Could you check a few things on this model? Use its own coordinates, in mm. Face numbers are marked on the shaded views. A direction names the side the tool comes from. Give positions to 0.01 mm unless a question says otherwise; leave off trailing zeros. Write each loop counter-clockwise with the first axis right and the second up, starting at its lowest first coordinate (ties: lowest second). Pieces come first, ordered by that corner, then holes. Notation, with made-up numbers: M 70.25,75 L 102.25,75 A8 ccw 102.25,86 Z; hole C 10.25,-32 d10. An arc over 180 degrees is marked long. One line per item, written item: value.
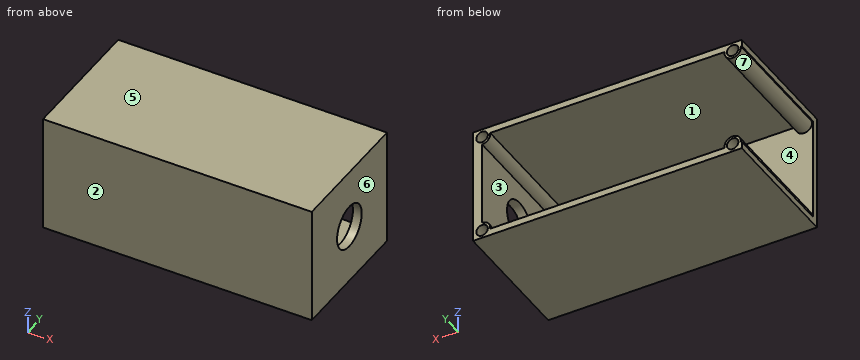
```python
from build123d import *

# Parameters (mm, degrees)
SKETCH1_W                 = 59.28
SKETCH1_H                 = 26
BOSS_EXTRUDE2_DEPTH       = 29
SKETCH3_W                 = 57.28
SKETCH3_H                 = 23
CUT_EXTRUDE1_DEPTH        = 27.5
SKETCH4_R                 = 4.75
SKETCH5_R                 = 4.8654
SKETCH9_R                 = 1.8
BOSS_EXTRUDE4_DEPTH       = 27.5
F_2_0MM_DOWEL_HOLE3_D     = 2.54
F_2_0MM_DOWEL_HOLE3_DEPTH = 10
MIRROR2_COPY_1_SKETCH_R   = 1.8
MIRROR2_COPY_1_DEPTH      = 27.5
MIRROR2_COPY_2_D          = 2.54
MIRROR2_COPY_2_DEPTH      = 10


with BuildPart() as part:
    # Sketch1 → Boss-Extrude2 (new body)
    with BuildSketch(Plane(origin=(0, 0, 0), x_dir=(1, 0, 0), z_dir=(0, 1, 0))):
        with Locations((29.64, 13)):
            Rectangle(SKETCH1_W, SKETCH1_H)
    extrude(amount=BOSS_EXTRUDE2_DEPTH)

    # Sketch3 → Cut-Extrude1 (cut)
    with BuildSketch(Plane(origin=(0, 29, 0), x_dir=(1, 0, 0), z_dir=(0, 1, 0))):
        with Locations((28.64, 13)):
            Rectangle(SKETCH3_W, SKETCH3_H)
    extrude(amount=-CUT_EXTRUDE1_DEPTH, mode=Mode.SUBTRACT)

    # Sketch4 → Cut-Loft1 section 0
    with BuildSketch(Plane(origin=(59.28, 0, 0), x_dir=(0, 0, -1), z_dir=(1, 0, 0))):
        with Locations((13, 14.5)):
            Circle(SKETCH4_R)
    # Sketch5 → Cut-Loft1 section 1
    with BuildSketch(Plane.ZY.offset(-57.28)):
        with Locations((-13, 14.5)):
            Circle(SKETCH5_R)
    loft(mode=Mode.SUBTRACT)

    # Sketch9 → Boss-Extrude4 (add)
    with BuildSketch(Plane(origin=(0, 29, 0), x_dir=(1, 0, 0), z_dir=(0, 1, 0))):
        with Locations((57.28, 1.8)):
            Circle(SKETCH9_R)
    boss_extrude4 = extrude(amount=-BOSS_EXTRUDE4_DEPTH)

    # Ø2.0mm Dowel Hole3
    with Locations(Plane(origin=(0, 29, 0), x_dir=(1, 0, 0), z_dir=(0, 1, 0))):
        with Locations((57.28, 1.8)):
            f_2_0mm_dowel_hole3 = Hole(F_2_0MM_DOWEL_HOLE3_D / 2, depth=F_2_0MM_DOWEL_HOLE3_DEPTH)

    # Mirror1: Boss-Extrude4, Ø2.0mm Dowel Hole3 across plane
    add(boss_extrude4.mirror(Plane(origin=(0, 0, -13), x_dir=(1, 0, 0), z_dir=(0, 0, -1))))
    add(f_2_0mm_dowel_hole3.mirror(Plane(origin=(0, 0, -13), x_dir=(1, 0, 0), z_dir=(0, 0, -1))), mode=Mode.SUBTRACT)

    # Mirror2: Boss-Extrude4, Ø2.0mm Dowel Hole3 across plane
    add(boss_extrude4.mirror(Plane.ZY.offset(-29.64)))
    add(f_2_0mm_dowel_hole3.mirror(Plane.ZY.offset(-29.64)), mode=Mode.SUBTRACT)

    # Mirror2 copy 1 sketch → Mirror2 copy 1 (add)
    with BuildSketch(Plane(origin=(59.28, 29, -26), x_dir=(-1, 0, 0), z_dir=(0, 1, 0))):
        with Locations((57.28, 1.8)):
            Circle(MIRROR2_COPY_1_SKETCH_R)
    extrude(amount=-MIRROR2_COPY_1_DEPTH)

    # Mirror2 copy 2
    with Locations(Plane(origin=(59.28, 29, -26), x_dir=(-1, 0, 0), z_dir=(0, 1, 0))):
        with Locations((57.28, 1.8)):
            Hole(MIRROR2_COPY_2_D / 2, depth=MIRROR2_COPY_2_DEPTH)


solid = part.part
```
1) Please list where these lines run through material, in increasing order: L1, parallel to Z at x = 11, y = 17; L2, parallel to Y at x = 52.5, z = -16.5; L3, parallel to X at y = 10.5, z = -17. Write a range as from..to.
Outcome:
L1: z = -26..-24.5, -1.5..0
L2: y = 0..1.5
L3: x = 57.28..59.28
2) If we section it at A-A, the plane z = -13: Write out the boundary of the cut face in (x, y), then the cut area to 3 significant figures.
Outcome:
outline: M 0,0 L 59.28,0 L 59.28,9.75 L 57.28,9.63 L 57.28,1.5 L 0,1.5 Z; M 57.28,19.37 L 59.28,19.25 L 59.28,29 L 57.28,29 Z
area: 125 mm^2
3) On a 3-axis mill with a long thin cutter (end or side, diameter ignored), from which of +Z, -Z, +X, -X, +Y, -Y can I reach the whole of each face in a straight line? I mean the marked faces 1, 2 and 3. Say none if no direction works.
Outcome:
face 1: +Y
face 2: +Z, -Z, +X, -X, -Y
face 3: -X, +Y
4) We'd pull the mould along X, two halves only. Please class the marked faces 4, 5, 6 and 7: pulls with the +X half, pulls with the -X half, needs draft (parallel to the pull), parting line crosses it, or undercut.
Outcome:
face 4: undercut
face 5: needs draft
face 6: pulls with the +X half
face 7: undercut
5) If we section it at B-B, the plane y = 23.5: Write out the boundary of the cut face in (x, z).
Outcome:
outline: M 0,-26 L 59.28,-26 L 59.28,0 L 0,0 L 0,-1.5 L 0.23,-1.5 A1.8 ccw long 3.77,-1.5 L 55.51,-1.5 A1.8 ccw 57.28,-3.6 L 57.28,-22.4 A1.8 ccw 55.51,-24.5 L 3.77,-24.5 A1.8 ccw long 0.23,-24.5 L 0,-24.5 Z; hole C 2,-24.2 d2.54; hole C 2,-1.8 d2.54; hole C 57.28,-24.2 d2.54; hole C 57.28,-1.8 d2.54
6) If we section it at D-D, the plane x = 4.5: Write out the boundary of the cut face in (y, z), then the cut area to 4 significant figures.
Outcome:
outline: M 0,-26 L 29,-26 L 29,-24.5 L 1.5,-24.5 L 1.5,-1.5 L 29,-1.5 L 29,0 L 0,0 Z
area: 121.5 mm^2
7) If we section it at C-C, the plane y = 7.75: Write out the boundary of the cut face in (x, z), then the cut area to 3 significant figures.
Outcome:
outline: M 0,-26 L 59.28,-26 L 59.28,0 L 0,0 L 0,-1.5 L 0.23,-1.5 A1.8 ccw long 3.77,-1.5 L 55.51,-1.5 A1.8 ccw 57.28,-3.6 L 57.28,-22.4 A1.8 ccw 55.51,-24.5 L 3.77,-24.5 A1.8 ccw long 0.23,-24.5 L 0,-24.5 Z
area: 242 mm^2
8) I'm going to push flat-ended pins straight in: pin 1 (8 mm diameter, centred on y = 7, z = -16, fed in from -X); pin 2 (0.8 mm diameter, centred on x = 57.5, z = -1.5, fed in from +Y); pin 3 (7 mm diameter, centred on x = 41, z = -9.5, fed in from +Y). Where does each tip first touch, or does it pass through?
Outcome:
pin 1: stops at x = 57.28
pin 2: stops at y = 19
pin 3: stops at y = 1.5
